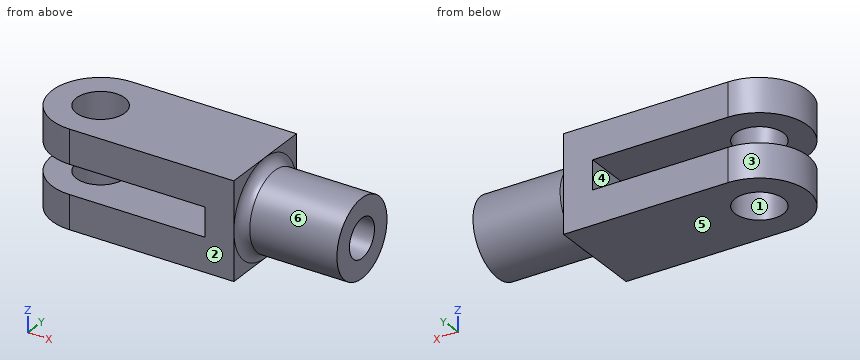
from build123d import *

# Parameters (mm, degrees)
SKETCH1_R               = 2.5
BOSS_EXTRUDE1_DEPTH     = 5
CUT_EXTRUDE1_DEPTH      = 19.41195264
CUT_EXTRUDE1_DEPTH_BACK = 19.41195264
SKETCH2_W               = 19
SKETCH2_H               = 3
SKETCH3_R               = 4
SKETCH3_R_2             = 2
BOSS_EXTRUDE2_DEPTH     = 10
FILLET1_R               = 1


with BuildPart() as part:
    # Sketch1 → Boss-Extrude1 (new, symmetric)
    with BuildSketch(Plane.XY):
        with BuildLine():
            ThreePointArc((0, -5), (-5, 0), (0, 5))
            Line((0, 5), (17, 5))
            Line((17, 5), (17, -5))
            Line((17, -5), (0, -5))
        make_face()
        Circle(SKETCH1_R, mode=Mode.SUBTRACT)
    extrude(amount=BOSS_EXTRUDE1_DEPTH, both=True)

    # Sketch2 → Cut-Extrude1 (cut, two sides: drawn at the far end of the back side and taken through both)
    with BuildSketch(Plane(origin=(0, 0, 0), x_dir=(1, 0, 0), z_dir=(0, 1, 0)).offset(-CUT_EXTRUDE1_DEPTH_BACK)):
        with Locations((4.5, 0)):
            Rectangle(SKETCH2_W, SKETCH2_H)
    extrude(amount=CUT_EXTRUDE1_DEPTH + CUT_EXTRUDE1_DEPTH_BACK, mode=Mode.SUBTRACT)

    # Sketch3 → Boss-Extrude2 (add)
    with BuildSketch(Plane(origin=(17, 0, 0), x_dir=(0, 0, -1), z_dir=(1, 0, 0))):
        Circle(SKETCH3_R)
        Circle(SKETCH3_R_2, mode=Mode.SUBTRACT)
    extrude(amount=BOSS_EXTRUDE2_DEPTH)

    # Fillet1
    fillet1_edges = [part.edges().sort_by_distance(p)[0] for p in [
        (17, 0, 4),
    ]]
    fillet(fillet1_edges, radius=FILLET1_R - 0.0001)  # a hair under: the kernel refuses the full size


solid = part.part
Geometry check sheet. Reference: the model listing, model coordinates, mm. Face numbers are marked on the shaded views. A direction names the side the tool comes from. Give positions to 0.01 mm unless a question says otherwise; leave off trailing zeros. Order: outer loops, then holes, each group sorted by start corner. A loop starts at its lowest first (then second) coordinate and runs counter-clockwise, first axis right, second up.
1. Scan lines: line 1 (Y direction, x = 23.25, z = 0); line 2 (Z direction, x = 10.5, y = -1.5); line 3 (Y direction, x = 0, z = -2.5). Record each from-to range of solid material in increasing order.
Completed:
line 1: y = -4 to -2, 2 to 4
line 2: z = -5 to -1.5, 1.5 to 5
line 3: y = -5 to -2.5, 2.5 to 5
2. Draft check along X on the marked faces 1, 2 and 3. Enter one of: pulls with the +X half, pulls with the -X half, needs draft (parallel to the pull), parting line crosses it, or undercut.
Completed:
face 1: undercut
face 2: needs draft
face 3: pulls with the -X half
3. Depth check by flat-ended pin: pin 1 (1 mm diameter, centred on x = 18.5, y = -1, fed in from +Z); pin 2 (3 mm diameter, centred on x = 0, y = 0, fed in from -Z); pin 3 (0.9 mm diameter, centred on y = 0, z = 0, fed in from -X). Enter the tip coordinate at first touch or a pass-through.
Completed:
pin 1: stops at z = 3.97
pin 2: passes through
pin 3: stops at x = 14
4. Sectioned sample at D-D (x = 21). Record the boundary of the cut face in (y, z), then the cut area to 3 significant figures.
Completed:
outline: circle Ø8 at (0, 0); hole circle Ø4 at (0, 0)
area: 37.7 mm2
5. Sectioned sample at A-A (x = 3). Record the boundary of the cut face in (y, z), then the cut area to 3 significant figures.
Completed:
outline: (-5, -5) - (5, -5) - (5, -1.5) - (-5, -1.5) - close; (-5, 1.5) - (5, 1.5) - (5, 5) - (-5, 5) - close
area: 70.0 mm2
6. Access from +Z, -Z, +X, -X, +Y, -Y to the whole of each face (thin tool, end or side, straight path). Record for the marked faces 4, 5 and 6.
Completed:
face 4: -X, +Y, -Y
face 5: -Z, +X, -X, +Y, -Y
face 6: +X
7. Sectioned sample at B-B (y = 0). State how many separate pieces and enclosed holes the cut face has, then the cut area to 3 significant figures.
Completed:
separate pieces: 3
enclosed holes: 0
area: 168 mm2
